The figure shows three views and two pictorial views of one solid part (mm, origin at its lowest corner). Answer the questions. Round coordinates to 2 decimals unless told otherwise and drop trailing zeros. Loops run counter-clockwise (first coordinate to the right, second up) from the corner with the lowest first, then second, coordinate; pieces in that order, holes last. Notation, with made-up numbers: (17.25, -9.75) -> (60.25, -9.75) arc R7 ccw to (60.25, -4.75) -> close; hole circle Ø9 at (-29.75, -2). An arc over 180 degrees is marked (long way). Put each result on its own line as item: value.
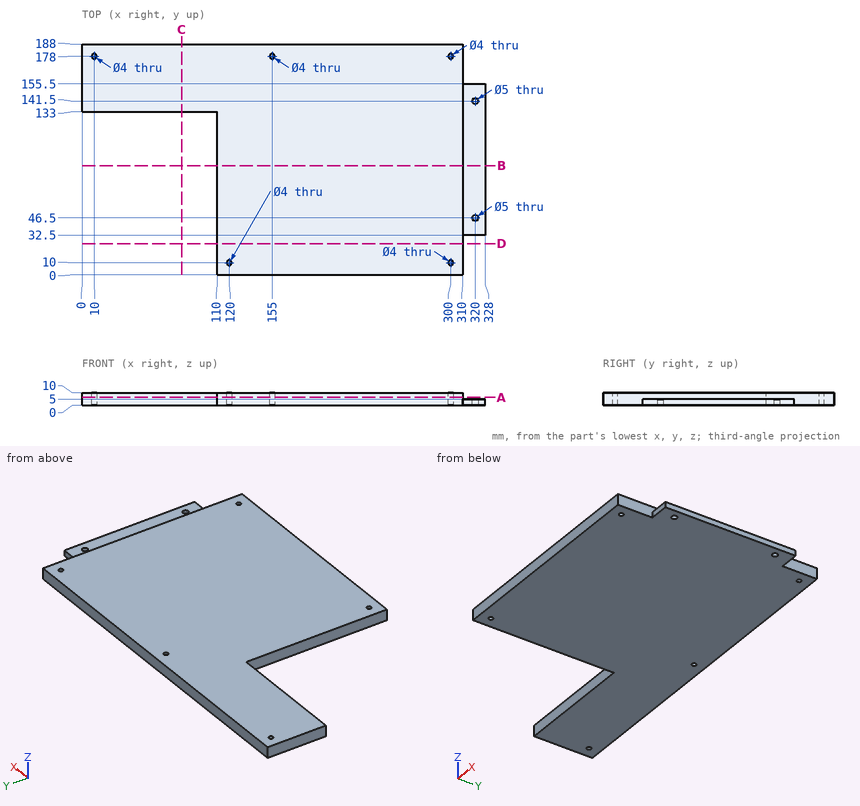
Item 1: Find the intervals of material crossed by line 1 along Y through (x, z) = (300, 7.25); line 2 along X through (y, z) = (178, 5.5); line 3 along Y through (x, z) = (320, 3.7), in increasing order.
Derived:
line 1: y = 0 to 8, 12 to 176, 180 to 188
line 2: x = 0 to 8, 12 to 153, 157 to 298, 302 to 310
line 3: y = 32.5 to 44, 49 to 139, 144 to 155.5
Item 2: Flat-ended cylindrical pins translate along their axes: pin 1 Ø5 at (x, y) = (10, 178) entering from +Z; pin 2 Ø5 at (y, z) = (45.5, 4) entering from -X; pin 3 Ø1.5 at (x, z) = (318, 1.5) entering from +Y; pin 4 Ø3 at (x, z) = (79, 5.5) entering from -Y. Find the tip coordinate at first contact, or state that the pin passes through.
Derived:
pin 1: stops at z = 10
pin 2: stops at x = 110
pin 3: stops at y = 155.5
pin 4: stops at y = 133
Item 3: The part is cut by section C-C (x = 81). Determine the outline of the cut face in (y, z), then the cut area to 3 significant figures.
Derived:
outline: (133, 0) -> (188, 0) -> (188, 10) -> (133, 10) -> close
area: 550 mm^2
Item 4: The part is cut by section D-D (y = 25.5). Determine the outline of the cut face in (x, z), then the cut area to 3 significant figures.
Derived:
outline: (110, 0) -> (310, 0) -> (310, 10) -> (110, 10) -> close
area: 2,000 mm^2
Item 5: The part is cut by section B-B (y = 89). Determine the outline of the cut face in (x, z).
Derived:
outline: (110, 0) -> (328, 0) -> (328, 5) -> (310, 5) -> (310, 10) -> (110, 10) -> close
Item 6: The part is cut by section A-A (z = 6.5). Determine the outline of the cut face in (x, y).
Derived:
outline: (0, 133) -> (110, 133) -> (110, 0) -> (310, 0) -> (310, 188) -> (0, 188) -> close; hole circle Ø4 at (10, 178); hole circle Ø4 at (120, 10); hole circle Ø4 at (155, 178); hole circle Ø4 at (300, 10); hole circle Ø4 at (300, 178)
